Part model, mm, in its own coordinate system. Face numbers are marked on the shaded views. A direction names the side the tool comes from. Round coordinates to 2 decimals unless told otherwise and drop trailing zeros. Loops run counter-clockwise (first coordinate to the right, second up) from the corner with the lowest first, then second, coordinate; pieces in that order, holes last. Notation, with made-up numbers: M -17.5,56.25 L 9.5,56.25 A14 cw 9.5,81.25 Z; hole C 87.25,12 d5. An arc over 180 degrees is marked long. Put each result on its own line as item: value. Start each with the question number.
1) Slice it at B-B on x = 218. Give the cut face in (y, z), then the cut area to 3 significant figures.
2) Slice it at D-D on x = 116. Give the cut face in (y, z).
3) Probe line 1 along X through (y, z) = (39, 69); line 2 along Z through (x, y) = (60.5, 47); line 3 along Y through (x, z) = (97, 64.5). List the from-to ranges inside material, lowest first.
4) Pull direction Z, two halves, no side cores. Call the marked faces 6, 7 and 8: +Z half, -Z half, draft (parallel to the pull), parting line (faces both ways), or undercut.
5) Drop flat-ended pins along their axis: pin 1 Ø12 at (x, y) = (44.5, 31) entering from -Z; pin 2 Ø10.5 at (x, z) = (151, -95.5) entering from +Y; pin 3 Ø25 at (y, z) = (88, 6) entering from -X; pin 4 Ø2 at (x, y) = (20, 11) entering from +Z. Give the stop position or say it passes through.
6) Which spindle directions (+Z, -Z, +X, -X, +Y, -Y) get a long thin tool onto all of the face, cutting with end or side? Do the marked faces 1, 2, 3, 4 and 5. Say none if no direction does.
7) Slice it at C-C on y = 25. Give the cut face in (x, z).
8) Slice it at A-A on z = 0. Give the cut face in (x, y), then the cut area to 3 significant figures.
```python
from build123d import *

# Parameters (mm, degrees)
BOSS_EXTRUDE2_DEPTH             = 75
CUT_EXTRUDE1_START              = -35
SKETCH3_W                       = 50
SKETCH3_H                       = 50
CUT_EXTRUDE1_DEPTH              = 165
SKETCH4_R                       = 14
BOSS_EXTRUDE3_DEPTH             = 5
CUT_EXTRUDE2_REACH              = 257
SKETCH5_R                       = 6
CUT_EXTRUDE2_DIRECTION_2_DEPTH  = 1
CUT_EXTRUDE4_REACH              = 257
SKETCH9_R                       = 8
FILLET2_R                       = 3
M6X1_0_TAPPED_HOLE2_D           = 5
M6X1_0_TAPPED_HOLE2_DEPTH       = 17.097848452
M6X1_0_TAPPED_HOLE2_CSINK_D     = 6.05
M6X1_0_TAPPED_HOLE2_CSINK_ANGLE = 90
M6X1_0_TAPPED_HOLE2_TIP         = 1.502151548
M3X0_5_TAPPED_HOLE1_D           = 2.5
M3X0_5_TAPPED_HOLE1_DEPTH       = 8.748924226
M3X0_5_TAPPED_HOLE1_CSINK_D     = 3.05
M3X0_5_TAPPED_HOLE1_CSINK_ANGLE = 90
M3X0_5_TAPPED_HOLE1_TIP         = 0.751075774
BOSS_EXTRUDE4_DEPTH             = 10
CUT_EXTRUDE5_START              = -11
SKETCH17_R                      = 7.75
CUT_EXTRUDE5_DEPTH              = 112
FILLET3_R                       = 10
FILLET4_R                       = 10


with BuildPart() as part:
    # Sketch1 → Boss-Extrude2 (new body, symmetric)
    with BuildSketch(Plane.XY):
        Polygon((0, 0), (250, 0), (250, 110), (208, 110), (208, 60), (200, 60), (200, 50), (0, 50), align=None)
    extrude(amount=BOSS_EXTRUDE2_DEPTH, both=True)

    # Sketch3 → Cut-Extrude1 (cut)
    with BuildSketch(Plane.ZY.offset(CUT_EXTRUDE1_START)):
        with Locations((0, 25)):
            Rectangle(SKETCH3_W, SKETCH3_H)
    extrude(amount=-CUT_EXTRUDE1_DEPTH, mode=Mode.SUBTRACT)

    # Sketch4 → Boss-Extrude3 (add)
    with BuildSketch(Plane.ZY):
        with Locations((0, 25)):
            Circle(SKETCH4_R)
    extrude(amount=BOSS_EXTRUDE3_DEPTH)

    # Sketch5 → Cut-Extrude2 (cut, up to next)
    with BuildSketch(Plane(origin=(250, 0, 0), x_dir=(0, 0, -1), z_dir=(1, 0, 0)), mode=Mode.PRIVATE) as cut_extrude2_sk1:
        with Locations((0, 25)):
            Circle(SKETCH5_R)
    cut_extrude2_tool1 = extrude(cut_extrude2_sk1.sketch, amount=-CUT_EXTRUDE2_REACH, mode=Mode.PRIVATE) & part.part
    add(cut_extrude2_tool1.solids().sort_by_distance((250, 25, 0))[0], mode=Mode.SUBTRACT)

    # Sketch5 → Cut-Extrude2 direction 2 (cut)
    with BuildSketch(Plane(origin=(250, 0, 0), x_dir=(0, 0, -1), z_dir=(1, 0, 0))):
        with Locations((0, 25)):
            Circle(SKETCH5_R)
    extrude(amount=CUT_EXTRUDE2_DIRECTION_2_DEPTH, mode=Mode.SUBTRACT)

    # Sketch9 → Cut-Extrude4 (cut, up to next)
    with BuildSketch(Plane.ZY.offset(5), mode=Mode.PRIVATE) as cut_extrude4_sk1:
        with Locations((0, 25)):
            Circle(SKETCH9_R)
    cut_extrude4_tool1 = extrude(cut_extrude4_sk1.sketch, amount=-CUT_EXTRUDE4_REACH, mode=Mode.PRIVATE) & part.part
    add(cut_extrude4_tool1.solids().sort_by_distance((-5, 25, 0))[0], mode=Mode.SUBTRACT)

    # Fillet2
    fillet2_edges = [part.edges().sort_by_distance(p)[0] for p in [
        (0, 25, -14),
    ]]
    fillet(fillet2_edges, radius=FILLET2_R)

    # M6x1.0 Tapped Hole2
    with Locations(Plane(origin=(208, 85, -45), x_dir=(0, 0, -1), z_dir=(-1, 0, 0))):
        with Locations((0, 0), (-90, 0)):
            CounterSinkHole(M6X1_0_TAPPED_HOLE2_D / 2, M6X1_0_TAPPED_HOLE2_CSINK_D / 2, depth=M6X1_0_TAPPED_HOLE2_DEPTH, counter_sink_angle=M6X1_0_TAPPED_HOLE2_CSINK_ANGLE)
            with Locations((0, 0, -(M6X1_0_TAPPED_HOLE2_DEPTH + M6X1_0_TAPPED_HOLE2_TIP / 2))):  # 118° drill point
                Cone(0, M6X1_0_TAPPED_HOLE2_D / 2, M6X1_0_TAPPED_HOLE2_TIP, mode=Mode.SUBTRACT)

    # M3x0.5 Tapped Hole1
    with Locations(Plane(origin=(20, 39, 75), x_dir=(1, 0, 0), z_dir=(0, 0, 1))):
        with Locations((0, 0), (68, 0), (68, -28), (0, -28)):
            CounterSinkHole(M3X0_5_TAPPED_HOLE1_D / 2, M3X0_5_TAPPED_HOLE1_CSINK_D / 2, depth=M3X0_5_TAPPED_HOLE1_DEPTH, counter_sink_angle=M3X0_5_TAPPED_HOLE1_CSINK_ANGLE)
            with Locations((0, 0, -(M3X0_5_TAPPED_HOLE1_DEPTH + M3X0_5_TAPPED_HOLE1_TIP / 2))):  # 118° drill point
                Cone(0, M3X0_5_TAPPED_HOLE1_D / 2, M3X0_5_TAPPED_HOLE1_TIP, mode=Mode.SUBTRACT)

    # Sketch15 → Boss-Extrude4 (add)
    with BuildSketch(Plane(origin=(0, 0, 0), x_dir=(1, 0, 0), z_dir=(0, 1, 0))):
        Polygon((127.240686807, -75), (172.759313193, -75), (165, -110), (135, -110), align=None)
    boss_extrude4 = extrude(amount=BOSS_EXTRUDE4_DEPTH)

    # Sketch17 → Cut-Extrude5 (cut)
    with BuildSketch(Plane(origin=(0, 10, 0), x_dir=(1, 0, 0), z_dir=(0, 1, 0)).offset(CUT_EXTRUDE5_START)):
        with Locations((150, -95)):
            Circle(SKETCH17_R)
    cut_extrude5 = extrude(amount=CUT_EXTRUDE5_DEPTH, mode=Mode.SUBTRACT)

    # Fillet3
    fillet3_edges = [part.edges().sort_by_distance(p)[0] for p in [
        (135, 5, 110),
        (165, 5, 110),
        (172.759313193, 5, 75),
        (127.240686807, 5, 75),
    ]]
    fillet(fillet3_edges, radius=FILLET3_R)

    # Mirror3: Boss-Extrude4, Cut-Extrude5 across plane
    add(boss_extrude4.mirror(Plane.XY))
    add(cut_extrude5.mirror(Plane.XY), mode=Mode.SUBTRACT)

    # Fillet4
    fillet4_edges = [part.edges().sort_by_distance(p)[0] for p in [
        (165, 5, -110),
        (135, 5, -110),
        (127.240686807, 5, -75),
        (172.759313193, 5, -75),
    ]]
    fillet(fillet4_edges, radius=FILLET4_R)


solid = part.part
```
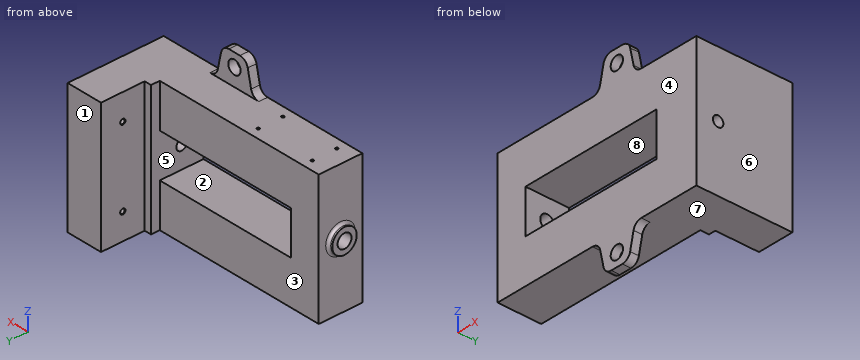
Recorded:
1. outline: M 0,-75 L 110,-75 L 110,75 L 0,75 Z; hole C 25,0 d12; hole C 85,-45 d5; hole C 85,45 d5
1. area: 16,300 mm2
2. outline: M 0,-75 L 50,-75 L 50,-25 L 0,-25 Z; M 0,25 L 50,25 L 50,75 L 0,75 Z
3. line 1: x = 0 to 18.75, 21.25 to 86.75, 89.25 to 250
3. line 2: z = -75 to -25, 25 to 75
3. line 3: y = 0 to 50
4. face 6: draft
4. face 7: -Z half
4. face 8: undercut
5. pin 1: stops at z = -75
5. pin 2: passes through
5. pin 3: stops at x = 208
5. pin 4: stops at z = 66.1
6. face 1: +Z, -Z, +X, -X, +Y
6. face 2: +Y, -Y
6. face 3: +Z, -Z, -X, +Y
6. face 4: +Z, -Z, +X, -X, -Y
6. face 5: +Y
7. outline: M -5,-14 L -3,-14 A3 cw 0,-17 L 0,-75 L 250,-75 L 250,-6 L 200,-6 L 200,-25 L 35,-25 L 35,-8 L -5,-8 Z; M -5,8 L 35,8 L 35,25 L 200,25 L 200,6 L 250,6 L 250,75 L 0,75 L 0,17 A3 cw -3,14 L -5,14 Z
8. outline: M -5,11 L -3,11 A3 cw 0,8 L 0,0 L 35,0 L 35,17 L -5,17 Z; M -5,33 L 35,33 L 35,50 L 0,50 L 0,42 A3 cw -3,39 L -5,39 Z; M 200,0 L 250,0 L 250,19 L 200,19 Z; M 200,31 L 250,31 L 250,110 L 208,110 L 208,60 L 200,60 Z
8. area: 5,750 mm2
